The model under review builds one solid part; all positions refer to its coordinate system, in mm. Coordinates: 2 decimals unless noted, no trailing zeros. Loops run counter-clockwise (first coordinate to the right, second up) from the corner with the lowest first, then second, coordinate; pieces in that order, holes last. Notation, with made-up numbers: M 26,-7.5 L 31,-7.5 A21 cw 31,5.5 Z; hole C 3.25,-38.75 d2. An arc over 180 degrees is marked long. One line per item, written item: value.
```python
from build123d import *

# Parameters (mm, degrees)
SKETCH2_W             = 228.06
SKETCH2_H             = 20
BOSS_EXTRUDE1_DEPTH   = 3.175
F_6_CLEARANCE_HOLE1_D = 3.7973


with BuildPart() as part:
    # Sketch2 → Boss-Extrude1 (new body)
    with BuildSketch(Plane.XY):
        with Locations((114.03, 10)):
            Rectangle(SKETCH2_W, SKETCH2_H)
    extrude(amount=-BOSS_EXTRUDE1_DEPTH)

    # #6 Clearance Hole1 (through all)
    with Locations(Plane.XY):
        with Locations((218.06, 10), (39.475, 10)):
            Hole(F_6_CLEARANCE_HOLE1_D / 2)


solid = part.part
```
(1) To check wall thickness, follow L1, parallel to Y at x = 218.06, z = -1.85. State the ranges of the line that lie inside material, in increasing order. Write a range as [from, to].
Checks:
L1: [0, 8.1], [11.9, 20]
(2) Draft analysis for pull direction Y (two halves, no side actions). For faces 1 (the face through (112, 10, 0)), 2 (the face through (216.25, 10.57, -1.61)), state which applies: pulls with the +Y half, pulls with the -Y half, needs draft (parallel to the pull), parting line crosses it, or undercut.
Checks:
face 1: needs draft
face 2: undercut
(3) Add section B-B on y = 10. State the section outline as (x, z) points (3 decimals).
Checks:
outline: M 0,-3.175 L 37.576,-3.175 L 37.576,0 L 0,0 Z; M 41.374,-3.175 L 216.161,-3.175 L 216.161,0 L 41.374,0 Z; M 219.959,-3.175 L 228.06,-3.175 L 228.06,0 L 219.959,0 Z
(4) Add section A-A on x = 218.06. State the section outline as (y, z) points (3 decimals).
Checks:
outline: M 0,-3.175 L 8.101,-3.175 L 8.101,0 L 0,0 Z; M 11.899,-3.175 L 20,-3.175 L 20,0 L 11.899,0 Z
